Design review of the part built by this model. Coordinates are the model's own, in mm. Round coordinates to 2 decimals unless told otherwise and drop trailing zeros. Loops run counter-clockwise (first coordinate to the right, second up) from the corner with the lowest first, then second, coordinate; pieces in that order, holes last. Notation, with made-up numbers: (-12, 79.25) -> (46, 79.25) arc R24 cw to (46, 111.25) -> close; hole circle Ø1 at (-22.75, 12.25). An arc over 180 degrees is marked (long way). Answer as CSV lines item,"result". Start each with the question number.
(1) Take a section at C-C, the plane z = 0.45. Write out the cut boundary in (x, y), and give its area (3 significant figures).
(2) Take a section at D-D, the plane z = 1.2. Write out the cut boundary in (x, y), and give its area (3 significant figures).
(3) To check wall thickness, follow line 1 (Y direction, x = 0, z = 0.75); line 2 (Y direction, x = -4, z = 1.5); line 3 (Z direction, x = 2.5, y = 5). State the ranges of each line that lie inside material, in increasing order. Write a range as from..to.
(4) For P1, Ø6, axis at x = -3.5, y = 4.5, coming from the -Z side; P2, Ø1, axis at y = 1.5, z = 1, coming from the +X side, all flat-tipped, find the tip position at first contact; note any pin that passes through.
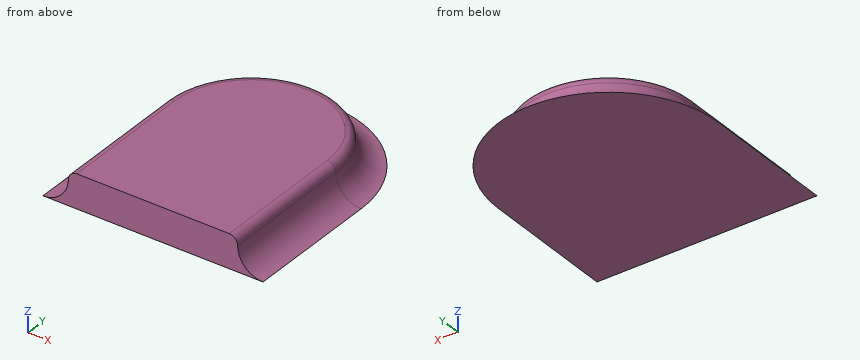
from build123d import *

# Parameters (mm, degrees)
EXTRUDE_1_DEPTH     = 2
SKETCH_2_W          = 17
SKETCH_2_H          = 17
EXTRUDE_2_DEPTH     = 5
FILLET_1_R          = 1.5
FILLET_2_R          = 0.5
SKETCH_3_W          = 5
SKETCH_3_H          = 17
CUT_EXTRUDE_4_DEPTH = 21.346989949


with BuildPart() as part:
    # 草图1 → 凸台-拉伸1 (new body)
    with BuildSketch(Plane.XY):
        with BuildLine():
            Line((-5, 0), (-5, -8))
            Line((-5, -8), (5, -8))
            Line((5, -8), (5, 0))
            ThreePointArc((5, 0), (0, 5), (-5, 0))
        make_face()
    extrude(amount=EXTRUDE_1_DEPTH)

    # 草图2 → 凸台-拉伸2 (add)
    with BuildSketch(Plane(origin=(0, 0, 0), x_dir=(-1, 0, 0), z_dir=(0, 0, -1))):
        with Locations((-1, -1.5)):
            Rectangle(SKETCH_2_W, SKETCH_2_H)
    extrude(amount=EXTRUDE_2_DEPTH)

    # 圆角1
    fillet_1_edges = [part.edges().sort_by_distance(p)[0] for p in [
        (5, -4, 0),
        (-5, -4, 0),
        (0, 5, 0),
    ]]
    fillet(fillet_1_edges, radius=FILLET_1_R)

    # 圆角2
    fillet_2_edges = [part.edges().sort_by_distance(p)[0] for p in [
        (5, -4, 2),
        (-5, -4, 2),
        (0, 5, 2),
    ]]
    fillet(fillet_2_edges, radius=FILLET_2_R - 0.0001)  # a hair under: the kernel refuses the full size

    # 草图3 → 切除-拉伸4 (cut, through all)
    with BuildSketch(Plane.ZY.offset(7.5)):
        with Locations((-2.5, -1.5)):
            Rectangle(SKETCH_3_W, SKETCH_3_H)
    extrude(amount=-CUT_EXTRUDE_4_DEPTH, mode=Mode.SUBTRACT)


solid = part.part
The answers:
1,outline,"(-5.43, -8) -> (5.43, -8) -> (5.43, 0) arc R5.43 ccw to (-5.43, 0) -> close"
1,area,"133 mm²"
2,outline,"(-5.03, -8) -> (5.03, -8) -> (5.03, 0) arc R5.03 ccw to (-5.03, 0) -> close"
2,area,"120 mm²"
3,line 1,"-8..5.2"
3,line 2,"-8..3"
3,line 3,"0..0.31"
4,P1,"z = 0"
4,P2,"x = 5.19"
